Verification items for the finished model (mm, model axes). A direction names the side the tool comes from. Round coordinates to 2 decimals unless told otherwise and drop trailing zeros. Loops run counter-clockwise (first coordinate to the right, second up) from the corner with the lowest first, then second, coordinate; pieces in that order, holes last. Notation, with made-up numbers: M 46,45 L 89,45 A22 ccw 89,53 Z; hole C 69,-24 d5. An arc over 180 degrees is marked long. Answer as CSV lines item,"result".
```python
from build123d import *

# Parameters (mm, degrees)
F0_R     = 3.81
F1_DEPTH = 17.78
F2_R     = 4.445
F3_DEPTH = 0.762
F4_SIZE  = 1.27


with BuildPart() as f1:
    # F0 (on Front) → F1 (new body)
    with BuildSketch(Plane.XZ):
        Circle(F0_R)
    extrude(amount=F1_DEPTH)

    # F2 (on Front) → F3 (join)
    with BuildSketch(Plane.XZ):
        Circle(F2_R)
    extrude(amount=-F3_DEPTH)

    # F4
    f4_edges = [f1.edges().sort_by_distance(p)[0] for p in [
        (-3.81, -17.78, 0),
    ]]
    chamfer(f4_edges, length=F4_SIZE)


solid = f1.part
```
1) Material ranges on probe 1 along Y at (x, z) = (2.5, 3); probe 2 along Y at (x, z) = (-3.25, -0.5); probe 3 along Z at (x, y) = (-0.75, -10.25), recorded low to high.
Here are the results:
probe 1,"y = 0 to 0.76"
probe 2,"y = -17.03 to 0.76"
probe 3,"z = -3.74 to 3.74"
2) Go/stop test with flat-tipped pins: pin 1 (2 mm diameter, centred on y = -11.5, z = 1, fed in from +X); pin 2 (1.5 mm diameter, centred on y = -11, z = 3, fed in from -X). Record where each tip stops, or that it passes through.
Here are the results:
pin 1,"stops at x = 3.81"
pin 2,"stops at x = -3.07"
3) Draft check along X on faces 3 (the cylindrical face through (-0.96, 0.38, -4.34)), 4 (the flat face through (0, 0.762, 0)). Enter one of: +X half, -X half, draft (parallel to the pull), parting line (faces both ways), or undercut.
Here are the results:
face 3,"parting line"
face 4,"draft"
4) Section check B-B (z = 0). Record the cut outline in (x, y) (3 decimals).
Here are the results:
outline,"M -4.445,0 L -3.81,0 L -3.81,-16.51 L -2.54,-17.78 L 2.54,-17.78 L 3.81,-16.51 L 3.81,0 L 4.445,0 L 4.445,0.762 L -4.445,0.762 Z"
5) Section check C-C (y = -16). Record the cut outline in (x, z).
Here are the results:
outline,"C 0,0 d7.62"
6) Set-up check for faces 1 (the flat face through (0, -17.78, 0)), 2 (the cylindrical face through (-0.83, -8.14, -3.72)): record each of +Z, -Z, +X, -X, +Y, -Y from which the full face is reachable in a straight line by a thin tool's end or side.
Here are the results:
face 1,"+Z, -Z, +X, -X, -Y"
face 2,"-Y"
7) Section check A-A (x = 0). Record the cut outline in (y, z) (3 decimals).
Here are the results:
outline,"M -17.78,-2.54 L -16.51,-3.81 L 0,-3.81 L 0,-4.445 L 0.762,-4.445 L 0.762,4.445 L 0,4.445 L 0,3.81 L -16.51,3.81 L -17.78,2.54 Z"
